Autodesk Inventor part; units mm, degrees
ref_plane "YZ Plane" through (0, 0, 0) normal (1, 0, 0) x (0, 1, 0)
ref_plane "XZ Plane" through (0, 0, 0) normal (0, 1, 0) x (-1, 0, 0)
ref_plane "XY Plane" through (0, 0, 0) normal (0, 0, 1) x (1, 0, 0)
sketch "スケッチ1" plane through (0, 0, 0) normal (0, 0, 1) x (1, 0, 0)
  circle A0 centre (0, 0) radius 2.75
  dimension "d0" = 5.5
extrude "押し出し1" add sketch "スケッチ1" along normal blind 2
fillet "フィレット1" radius 1 1 edges at (-2.75, 0, 2)
sketch "スケッチ2" plane through (0, 0, 0) normal (0, 0, -1) x (-1, 0, 0)
  circle A0 centre (0, 0) radius 1.5
  dimension "d4" = 3
extrude "押し出し2" add sketch "スケッチ2" along normal blind 20
thread "ねじ1"
properties part number "Screw" material "真鍮"
Design review of the part built by this model. Coordinates are the model's own, in mm. A direction names the side the tool comes from. Coordinates: 2 decimals unless noted, no trailing zeros. Order: outer loops, then holes, each group sorted by start corner. A loop starts at its lowest first (then second) coordinate and runs counter-clockwise, first axis right, second up.
1) Clearance check with flat-ended pins moving along their axes: pin 1 (2 mm diameter, centred on y = -0.5, z = -13, fed in from -X); pin 2 (1.5 mm diameter, centred on x = 2, z = -9.5, fed in from -Y). State where each tip first meets the part, or that it passes through.
2) Take a section at A-A, the plane x = 0. Give the boundary of the cut face in (y, z), and give its area (3 significant figures).
3) Wall thickness on line 1 along Z through (x, y) = (-1.6, 0.2); line 2 along Y through (x, z) = (-0.1, -5); line 3 along Z through (x, y) = (1.5, -1.85): over which ranges is each line inside the solid? List them lowest first.
4) For faces 1 (the cylindrical face through (1.5, -0.07, -9.86)), 2 (the flat face through (0, 0, 2)), list the 3-axis set-ups (+Z, -Z, +X, -X, +Y, -Y) from which the entire face can be reached by the end or side of a thin tool; tool diameter is ignored.
5) Take a section at C-C, the plane z = -16.75. Give the boundary of the cut face in (x, y).
Returned:
1. pin 1: stops at x = -1.5
1. pin 2: stops at y = -0.83
2. outline: (-2.75, 0) - (-1.5, 0) - (-1.5, -20) - (1.5, -20) - (1.5, 0) - (2.75, 0) - (2.75, 1) arc R1 ccw to (1.75, 2) - (-1.75, 2) arc R1 ccw to (-2.75, 1) - close
2. area: 70.6 mm2
3. line 1: z = 0 to 2
3. line 2: y = -1.5 to 1.5
3. line 3: z = 0 to 1.78
4. face 1: -Z
4. face 2: +Z, +X, -X, +Y, -Y
5. outline: circle Ø3 at (0, 0)
